Input: part model. Units: mm. Frame: model coordinates. Coordinates: 2 decimals unless noted, no trailing zeros. Order: outer loops, then holes, each group sorted by start corner. A loop starts at its lowest first (then second) coordinate and runs counter-clockwise, first axis right, second up.
from build123d import *

# Parameters (mm, degrees)
F0_R     = 140
F1_DEPTH = 20
F2_R     = 3.5
F3_DEPTH = 20.001
F5_DEPTH = 25


with BuildPart() as f1:
    # F0 (on Top) → F1 (new body)
    with BuildSketch(Plane.XY):
        Circle(F0_R)
    extrude(amount=F1_DEPTH)

    # F2 (on face) → F3 (cut, through all)
    with BuildSketch(Plane.XY.offset(20)):
        with Locations((-10, 0)):
            Circle(F2_R)
        with Locations((10, 0)):
            Circle(F2_R)
    extrude(amount=-F3_DEPTH, mode=Mode.SUBTRACT)

    # F4 (on face) → F5 (cut)
    with BuildSketch(Plane.XY.offset(20)):
        with BuildLine():
            ThreePointArc((-91.923882, 91.923882), (-91.035749, 92.803515), (-90.139199, 93.674569))
            ThreePointArc((-90.139199, 93.674569), (-93.691649, 93.691649), (-93.674569, 90.139199))
            ThreePointArc((-93.674569, 90.139199), (-92.803515, 91.035749), (-91.923882, 91.923882))
        make_face()
        with BuildLine():
            ThreePointArc((-89.423882, 91.923882), (-89.60961, 92.869475), (-90.139199, 93.674569))
            ThreePointArc((-90.139199, 93.674569), (-91.035749, 92.803515), (-91.923882, 91.923882))
            Line((-91.923882, 91.923882), (-90.156115, 90.156115))
            ThreePointArc((-90.156115, 90.156115), (-89.614183, 90.967173), (-89.423882, 91.923882))
        make_face()
        with BuildLine():
            ThreePointArc((-93.674569, 90.139199), (-91.911862, 89.42391), (-90.156115, 90.156115))
            Line((-90.156115, 90.156115), (-91.923882, 91.923882))
            ThreePointArc((-91.923882, 91.923882), (-92.803515, 91.035749), (-93.674569, 90.139199))
        make_face()
        with BuildLine():
            ThreePointArc((91.923882, 91.923882), (92.803515, 91.035749), (93.674569, 90.139199))
            ThreePointArc((93.674569, 90.139199), (94.228954, 90.95608), (94.423882, 91.923882))
            ThreePointArc((94.423882, 91.923882), (92.869475, 94.238153), (90.139199, 93.674569))
            ThreePointArc((90.139199, 93.674569), (91.035749, 92.803515), (91.923882, 91.923882))
        make_face()
        with BuildLine():
            Line((90.156115, 90.156115), (91.923882, 91.923882))
            ThreePointArc((91.923882, 91.923882), (91.035749, 92.803515), (90.139199, 93.674569))
            ThreePointArc((90.139199, 93.674569), (89.42391, 91.911862), (90.156115, 90.156115))
        make_face()
        with BuildLine():
            ThreePointArc((90.156115, 90.156115), (91.911862, 89.42391), (93.674569, 90.139199))
            ThreePointArc((93.674569, 90.139199), (92.803515, 91.035749), (91.923882, 91.923882))
            Line((91.923882, 91.923882), (90.156115, 90.156115))
        make_face()
        with BuildLine():
            ThreePointArc((-93.674569, -90.139199), (-93.691649, -93.691649), (-90.139199, -93.674569))
            ThreePointArc((-90.139199, -93.674569), (-91.035749, -92.803515), (-91.923882, -91.923882))
            ThreePointArc((-91.923882, -91.923882), (-92.803515, -91.035749), (-93.674569, -90.139199))
        make_face()
        with BuildLine():
            ThreePointArc((-89.423882, -91.923882), (-89.614183, -90.967173), (-90.156115, -90.156115))
            Line((-90.156115, -90.156115), (-91.923882, -91.923882))
            ThreePointArc((-91.923882, -91.923882), (-91.035749, -92.803515), (-90.139199, -93.674569))
            ThreePointArc((-90.139199, -93.674569), (-89.60961, -92.869475), (-89.423882, -91.923882))
        make_face()
        with BuildLine():
            Line((-91.923882, -91.923882), (-90.156115, -90.156115))
            ThreePointArc((-90.156115, -90.156115), (-91.911862, -89.42391), (-93.674569, -90.139199))
            ThreePointArc((-93.674569, -90.139199), (-92.803515, -91.035749), (-91.923882, -91.923882))
        make_face()
        with BuildLine():
            ThreePointArc((94.423882, -91.923882), (94.228954, -90.95608), (93.674569, -90.139199))
            ThreePointArc((93.674569, -90.139199), (92.803515, -91.035749), (91.923882, -91.923882))
            ThreePointArc((91.923882, -91.923882), (91.035749, -92.803515), (90.139199, -93.674569))
            ThreePointArc((90.139199, -93.674569), (92.869475, -94.238153), (94.423882, -91.923882))
        make_face()
        with BuildLine():
            ThreePointArc((90.139199, -93.674569), (91.035749, -92.803515), (91.923882, -91.923882))
            Line((91.923882, -91.923882), (90.156115, -90.156115))
            ThreePointArc((90.156115, -90.156115), (89.42391, -91.911862), (90.139199, -93.674569))
        make_face()
        with BuildLine():
            ThreePointArc((91.923882, -91.923882), (92.803515, -91.035749), (93.674569, -90.139199))
            ThreePointArc((93.674569, -90.139199), (91.911862, -89.42391), (90.156115, -90.156115))
            Line((90.156115, -90.156115), (91.923882, -91.923882))
        make_face()
    extrude(amount=-F5_DEPTH, mode=Mode.SUBTRACT)


solid = f1.part
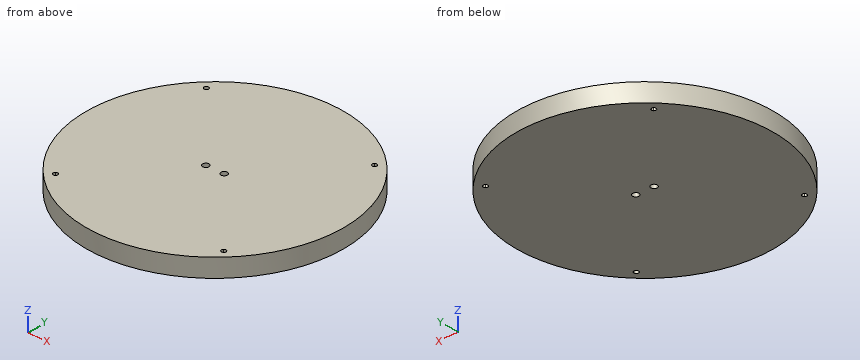
Item 1: Ray query, probe 1 along Y at (x, z) = (10, 7); probe 2 along X at (y, z) = (57, 13.5); probe 3 along Y at (x, z) = (31, 5.75). Return the intervals inside material, ascending.
Response values:
probe 1: y = -139.64 to -3.5, 3.5 to 139.64
probe 2: x = -127.87 to 127.87
probe 3: y = -136.52 to 136.52
Item 2: Cut plane A-A on z = 10. Return loops of the section in (x, y), then the cut area to 3 significant figures.
Response values:
outline: circle Ø280 at (0, 0); hole (-93.67, -90.14) arc R2.5 ccw (long way) to (-90.14, -93.67) arc R2.5 ccw to (-89.42, -91.92) arc R2.5 ccw to (-90.16, -90.16) arc R2.5 ccw to start; hole (-93.67, 90.14) arc R2.5 ccw to (-90.16, 90.16) arc R2.5 ccw to (-89.42, 91.92) arc R2.5 ccw to (-90.14, 93.67) arc R2.5 ccw (long way) to start; hole circle Ø7 at (-10, 0); hole circle Ø7 at (10, 0); hole (90.14, -93.67) arc R2.5 ccw to (94.42, -91.92) arc R2.5 ccw to (93.67, -90.14) arc R2.5 ccw to (90.16, -90.16) arc R2.5 ccw to start; hole (90.14, 93.67) arc R2.5 ccw to (90.16, 90.16) arc R2.5 ccw to (93.67, 90.14) arc R2.5 ccw to (94.42, 91.92) arc R2.5 ccw to start
area: 61,400 mm2
Item 3: Cut plane D-D on x = 102. Return loops of the section in (y, z), then the cut area to 3 significant figures.
Response values:
outline: (-95.9, 0) - (95.9, 0) - (95.9, 20) - (-95.9, 20) - close
area: 3,840 mm2
Item 4: Pin query (flat end, axial travel): pin 1 Ø5 at (x, z) = (-58, 17.5) entering from +Y; pin 2 Ø1.5 at (x, z) = (12.5, 11.5) entering from -Y; pin 3 Ø8 at (x, z) = (102, 15) entering from +Y. Return the tip coordinate at first contact, or that it passes through.
Response values:
pin 1: stops at y = 128.53
pin 2: stops at y = -139.51
pin 3: stops at y = 99.98
Item 5: Cut plane C-C on y = -48. Return loops of the section in (x, z), then the cut area to 3 significant figures.
Response values:
outline: (-131.51, 0) - (131.51, 0) - (131.51, 20) - (-131.51, 20) - close
area: 5,260 mm2
Item 6: Cut plane B-B on x = -10. Return loops of the section in (y, z).
Response values:
outline: (-139.64, 0) - (-3.5, 0) - (-3.5, 20) - (-139.64, 20) - close; (3.5, 0) - (139.64, 0) - (139.64, 20) - (3.5, 20) - close
